CAD build for the part. Positions are in the model's coordinates, mm. Face numbers are marked on the shaded views. Round coordinates to 2 decimals unless told otherwise and drop trailing zeros. Loops run counter-clockwise (first coordinate to the right, second up) from the corner with the lowest first, then second, coordinate; pieces in that order, holes last.
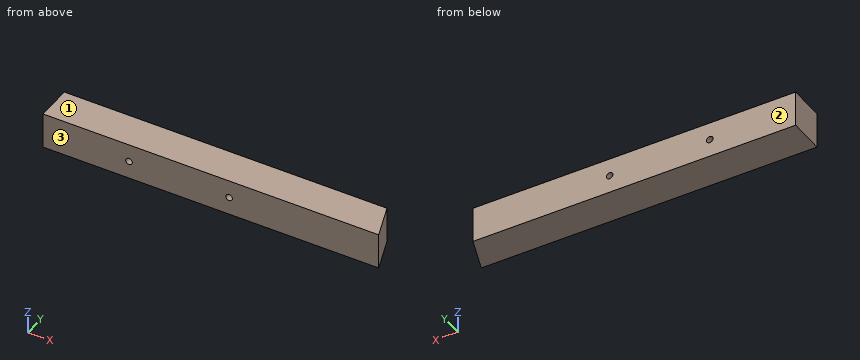
from build123d import *

# Parameters (mm, degrees)
SKETCH1_W               = 38.1
SKETCH1_H               = 38.1
BOSS_EXTRUDE1_DEPTH     = 355.6
CUT_EXTRUDE1_DEPTH      = 359.142251766
CUT_EXTRUDE2_DEPTH      = 359.142251766
CUT_EXTRUDE2_DEPTH_BACK = 359.142251766
SKETCH3_R               = 3.5


with BuildPart() as part:
    # Sketch1 → Boss-Extrude1 (new body)
    with BuildSketch(Plane(origin=(0, 0, 0), x_dir=(0, 0, -1), z_dir=(1, 0, 0))):
        Rectangle(SKETCH1_W, SKETCH1_H)
    extrude(amount=BOSS_EXTRUDE1_DEPTH)

    # Sketch2 → Cut-Extrude1 (cut, through all)
    with BuildSketch(Plane.XY.offset(19.05)):
        Polygon((355.6, -19.05), (341.890667107, 19.05), (355.6, 19.05), align=None)
    extrude(amount=-CUT_EXTRUDE1_DEPTH, mode=Mode.SUBTRACT)

    # Sketch3 → Cut-Extrude2 (cut, two sides: drawn at the far end of the back side and taken through both)
    with BuildSketch(Plane(origin=(0, -19.05, 0), x_dir=(-1, 0, 0), z_dir=(0, -1, 0)).offset(-CUT_EXTRUDE2_DEPTH_BACK)):
        with Locations(Location((-91.088392372, 0, 0), (0, 0, 90))):
            Circle(SKETCH3_R)
        with Locations(Location((-197.087368962, 0, 0), (0, 0, 90))):
            Circle(SKETCH3_R)
    extrude(amount=CUT_EXTRUDE2_DEPTH + CUT_EXTRUDE2_DEPTH_BACK, mode=Mode.SUBTRACT)


solid = part.part
Item 1: Mould opens along Y. For the marked faces 1, 2 and 3 say: released by +Y, released by -Y, zero draft, split by the parting line, or undercut.
Verdict:
face 1: zero draft
face 2: released by +Y
face 3: released by -Y
Item 2: Wall check: L1, parallel to X at y = -11, z = 0; L2, parallel to X at y = 5, z = 0; L3, parallel to X at y = 4, z = 8. Give the ranges that are in metal, low to high.
Verdict:
L1: x = 0 to 87.59, 94.59 to 193.59, 200.59 to 352.7
L2: x = 0 to 87.59, 94.59 to 193.59, 200.59 to 346.95
L3: x = 0 to 347.31
Item 3: Flat gauge pins, fed straight in: P1, Ø5.5, axis at x = 91.09, z = 0, coming from the +Y side; P2, Ø6, axis at y = 4.5, z = 12, coming from the -X side; P3, Ø12, axis at y = -10, z = 8, coming from the +X side. Where does each tip first touch, or does it go through?
Verdict:
P1: passes through
P2: stops at x = 0
P3: stops at x = 354.5
Item 4: Cut at A-A (z = 0). List the corners of the cut face in (x, y), plus the area to 3 significant figures.
Verdict:
outline: (0, -19.05) - (87.59, -19.05) - (87.59, 19.05) - (0, 19.05) - close; (94.59, -19.05) - (193.59, -19.05) - (193.59, 19.05) - (94.59, 19.05) - close; (200.59, -19.05) - (355.6, -19.05) - (341.89, 19.05) - (200.59, 19.05) - close
area: 12,800 mm2
Item 5: Cut at C-C (z = -13.5). List the corners of the cut face in (x, y).
Verdict:
outline: (0, -19.05) - (355.6, -19.05) - (341.89, 19.05) - (0, 19.05) - close
Item 6: Cut at B-B (y = 8). List the corners of the cut face in (x, z), plus the area to 3 significant figures.
Verdict:
outline: (0, -19.05) - (345.87, -19.05) - (345.87, 19.05) - (0, 19.05) - close; hole circle Ø7 at (91.09, 0); hole circle Ø7 at (197.09, 0)
area: 13,100 mm2
